Check sheet for the modelled part. Datum: model origin and axes. Units: mm. Round coordinates to 2 decimals unless told otherwise and drop trailing zeros. Order: outer loops, then holes, each group sorted by start corner. A loop starts at its lowest first (then second) coordinate and runs counter-clockwise, first axis right, second up.
Solid Edge part; units mm, degrees
sketch "Sketch1" plane through (0, 0, 0) normal (0, 0, 1) x (1, 0, 0)
  circle A0 centre (0, 0) radius 10.75
  line L0 (-22.9244, 24.7679) -> (22.9244, 24.7679)
  line L1 (22.9244, 24.7679) -> (22.9244, -24.7679)
  line L2 (22.9244, -24.7679) -> (-22.9244, -24.7679)
  line L3 (-22.9244, -24.7679) -> (-22.9244, 24.7679)
extrude "Protrusion1" add sketch "Sketch1" along normal blind 6
sketch "Sketch2" plane through (0, -24.7679, 3) normal (0, -1, 0) x (1, 0, 0)
  line L0 (-8.2053, 3) -> (-12.6053, 3)
  arc A0 (-8.2053, 3) -> (-12.6053, 3) centre (-10.4053, 3) cw
  line L1 (12.6053, 3) -> (8.2053, 3)
  arc A1 (12.6053, 3) -> (8.2053, 3) centre (10.4053, 3) cw
extrude "Cutout1" cut sketch "Sketch2" against normal through all
Item 1: Sectioned sample at A-A (x = 0). Record the cut outline in (y, z).
Answer:
outline: (-24.77, 0) - (-10.75, 0) - (-10.75, 6) - (-24.77, 6) - close; (10.75, 0) - (24.77, 0) - (24.77, 6) - (10.75, 6) - close
Item 2: Sectioned sample at D-D (y = 0). Record the cut outline in (x, z).
Answer:
outline: (-22.92, 0) - (-10.75, 0) - (-10.75, 3.83) arc R2.2 cw to (-12.61, 6) - (-22.92, 6) - close; (10.75, 0) - (22.92, 0) - (22.92, 6) - (12.61, 6) arc R2.2 cw to (10.75, 3.83) - close
Item 3: Release check for a two-part mould opening along X. For faces 1 (the cylindrical face through (-7.92, -7.27, 2.96)), 2 (the flat face through (-22.924, 0, 3)), 3 (the flat face through (22.924, 0, 3)), 4 (the flat face through (0, 11, 0)) record: released by +X, released by -X, zero draft, split by the parting line, or undercut.
Answer:
face 1: undercut
face 2: released by -X
face 3: released by +X
face 4: zero draft
Item 4: Scan lines: line 1 along Y through (x, z) = (0, 4.5); line 2 along X through (y, z) = (0, 1.5); line 3 along X through (y, z) = (-14, 4.5). Record each from-to range of solid material in increasing order.
Answer:
line 1: y = -24.77 to -10.75, 10.75 to 24.77
line 2: x = -22.92 to -10.75, 10.75 to 22.92
line 3: x = -22.92 to -12.01, -8.8 to 8.8, 12.01 to 22.92
Item 5: Sectioned sample at B-B (z = 1.5). Record the cut outline in (x, y), and give its area (3 significant figures).
Answer:
outline: (-22.92, -24.77) - (22.92, -24.77) - (22.92, 24.77) - (-22.92, 24.77) - close; hole circle Ø21.5 at (0, 0)
area: 1,910 mm2
Item 6: Sectioned sample at C-C (y = -13). Record the cut outline in (x, z), and give its area (3 significant figures).
Answer:
outline: (-22.92, 0) - (22.92, 0) - (22.92, 6) - (12.61, 6) arc R2.2 cw to (8.21, 6) - (-8.21, 6) arc R2.2 cw to (-12.61, 6) - (-22.92, 6) - close
area: 260 mm2
Item 7: Go/stop test with a flat-tipped pin: P1, Ø2, axis at x = 6.5, y = -7, coming from the +Z side. Record where the tip stops, or that it passes through.
Answer:
P1: passes through
